Part print with two shaded views. Sizes in mm from the minimum x, y, z corner. A direction names the side the tool comes from. Give positions to 0.01 mm unless a question says otherwise; leave off trailing zeros. Write each loop counter-clockwise with the first axis right and the second up, starting at its lowest first coordinate (ties: lowest second). Pieces come first, ordered by that corner, then holes.
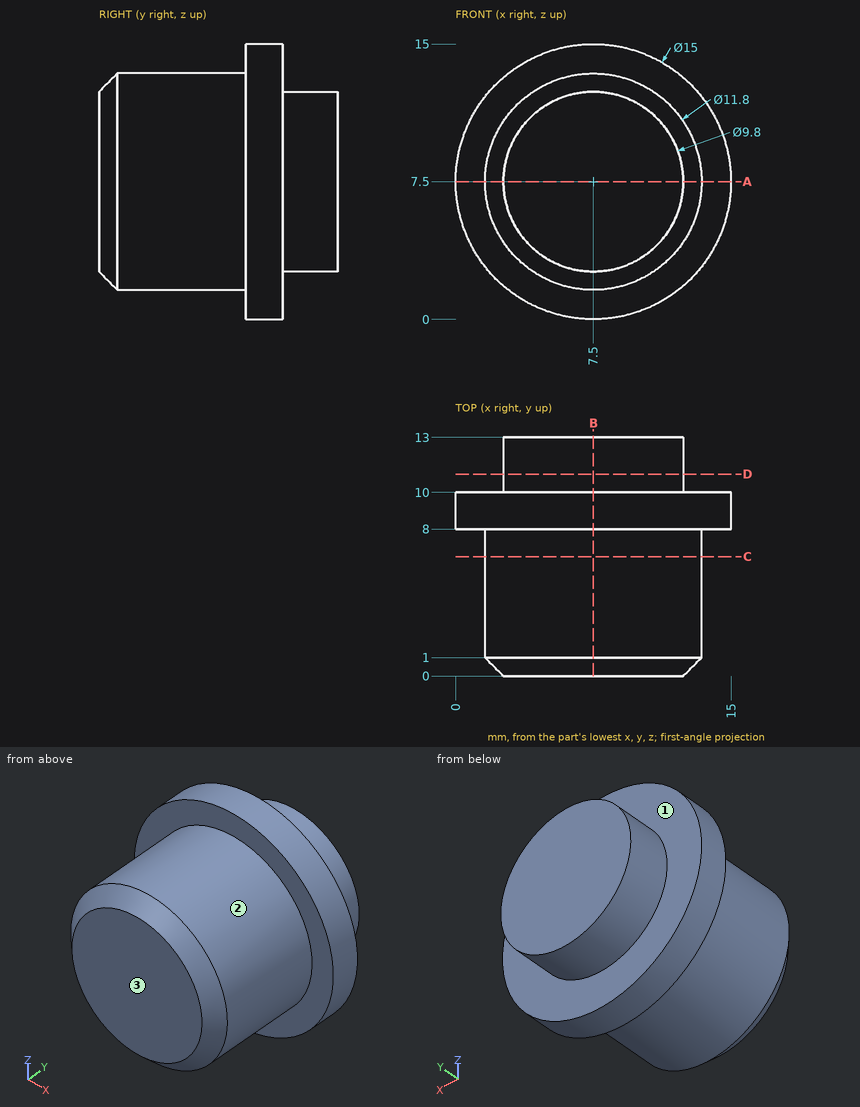
1) Saw through at D-D, the plane y = 11. Write the cut outline in (x, z), then the cut area to 3 significant figures.
Answers follow:
outline: circle Ø9.8 at (7.5, 7.5)
area: 75.4 mm2
2) Saw through at C-C, the plane y = 6.5. Write the cut outline in (x, z), then the cut area to 3 significant figures.
Answers follow:
outline: circle Ø11.8 at (7.5, 7.5)
area: 109 mm2
3) Saw through at B-B, the plane x = 7.5. Write the cut outline in (y, z), then the cut area to 3 significant figures.
Answers follow:
outline: (0, 2.6) - (1, 1.6) - (8, 1.6) - (8, 0) - (10, 0) - (10, 2.6) - (13, 2.6) - (13, 12.4) - (10, 12.4) - (10, 15) - (8, 15) - (8, 13.4) - (1, 13.4) - (0, 12.4) - close
area: 153 mm2
4) Saw through at A-A, the plane z = 7.5. Write the cut outline in (x, y).
Answers follow:
outline: (0, 8) - (1.6, 8) - (1.6, 1) - (2.6, 0) - (12.4, 0) - (13.4, 1) - (13.4, 8) - (15, 8) - (15, 10) - (12.4, 10) - (12.4, 13) - (2.6, 13) - (2.6, 10) - (0, 10) - close
5) Wall check: L1, parallel to Y at x = 12.5, z = 12.5; L2, parallel to Z at x = 7.25, y = 6.5; L3, parallel to X at y = 3.5, z = 11.5. Give the ranges that are in metal, low to high.
Answers follow:
L1: y = 8 to 10
L2: z = 1.61 to 13.39
L3: x = 3.16 to 11.84
6) 3-axis set-ups, long thin cutter, end or side, ignore diameter. For the marked faces 1, 2 and 3: which of +Z, -Z, +X, -X, +Y, -Y reach the whole face in a straight line?
Answers follow:
face 1: +Y
face 2: -Y
face 3: +Z, -Z, +X, -X, -Y
7) Pin check, flat tips, straight feed: pin 1 Ø6 at (y, z) = (9.5, 10.5) entering from +X; pin 2 Ø4 at (y, z) = (2.5, 5.5) entering from -X; pin 3 Ø6 at (x, y) = (12, 3.5) entering from +Z; pin 4 Ø1 at (x, z) = (4, 2.5) entering from +Y. Stop position of each tip, or through.
Answers follow:
pin 1: stops at x = 15
pin 2: stops at x = 1.6
pin 3: stops at z = 13.21
pin 4: stops at y = 10
